from build123d import *

# Parameters (mm, degrees)
SKETCH1_R               = 4.25
BOSS_EXTRUDE1_DEPTH     = 2
SKETCH1_3_R             = 7.25
SKETCH1_3_R_2           = 4.25
BOSS_EXTRUDE2_DEPTH     = 12
CUT_EXTRUDE1_DEPTH      = 47.818799643
CUT_EXTRUDE1_DEPTH_BACK = 47.818799643
SKETCH2_R               = 1.5


with BuildPart() as part:
    # Sketch1 → Boss-Extrude1 (new body)
    with BuildSketch(Plane(origin=(0, 0, 0), x_dir=(1, 0, 0), z_dir=(0, 1, 0))):
        with BuildLine():
            Line((6.579861092, 3.044327186), (24.395183951, 20.859650045))
            Line((24.395183951, 20.859650045), (20.859650045, 24.395183951))
            Line((20.859650045, 24.395183951), (3.044327186, 6.579861092))
            ThreePointArc((3.044327186, 6.579861092), (2.774454885, 6.698126611), (2.5, 6.805328794))
            Line((2.5, 6.805328794), (2.5, 32))
            Line((2.5, 32), (-2.5, 32))
            Line((-2.5, 32), (-2.5, 6.805328794))
            ThreePointArc((-2.5, 6.805328794), (-2.774454885, 6.698126611), (-3.044327186, 6.579861092))
            Line((-3.044327186, 6.579861092), (-20.859650045, 24.395183951))
            Line((-20.859650045, 24.395183951), (-24.395183951, 20.859650045))
            Line((-24.395183951, 20.859650045), (-6.579861092, 3.044327186))
            ThreePointArc((-6.579861092, 3.044327186), (-6.698126611, 2.774454885), (-6.805328794, 2.5))
            Line((-6.805328794, 2.5), (-32, 2.5))
            Line((-32, 2.5), (-32, -2.5))
            Line((-32, -2.5), (-6.805328794, -2.5))
            ThreePointArc((-6.805328794, -2.5), (-6.698126611, -2.774454885), (-6.579861092, -3.044327186))
            Line((-6.579861092, -3.044327186), (-24.395183951, -20.859650045))
            Line((-24.395183951, -20.859650045), (-20.859650045, -24.395183951))
            Line((-20.859650045, -24.395183951), (-3.044327186, -6.579861092))
            ThreePointArc((-3.044327186, -6.579861092), (-2.774454885, -6.698126611), (-2.5, -6.805328794))
            Line((-2.5, -6.805328794), (-2.5, -32))
            Line((-2.5, -32), (2.5, -32))
            Line((2.5, -32), (2.5, -6.805328794))
            ThreePointArc((2.5, -6.805328794), (2.774454885, -6.698126611), (3.044327186, -6.579861092))
            Line((3.044327186, -6.579861092), (20.859650045, -24.395183951))
            Line((20.859650045, -24.395183951), (24.395183951, -20.859650045))
            Line((24.395183951, -20.859650045), (6.579861092, -3.044327186))
            ThreePointArc((6.579861092, -3.044327186), (6.698126611, -2.774454885), (6.805328794, -2.5))
            Line((6.805328794, -2.5), (32, -2.5))
            Line((32, -2.5), (32, 2.5))
            Line((32, 2.5), (6.805328794, 2.5))
            ThreePointArc((6.805328794, 2.5), (6.698126611, 2.774454885), (6.579861092, 3.044327186))
        make_face()
        with Locations(Location((0, 0, 0), (0, 0, 270))):
            Circle(SKETCH1_R, mode=Mode.SUBTRACT)
    extrude(amount=BOSS_EXTRUDE1_DEPTH)

    # Sketch1_3 → Boss-Extrude2 (add)
    with BuildSketch(Plane(origin=(0, 0, 0), x_dir=(1, 0, 0), z_dir=(0, 1, 0))):
        with Locations(Location((0, 0, 0), (0, 0, 69.828728654))):
            Circle(SKETCH1_3_R)
        with Locations(Location((0, 0, 0), (0, 0, 270))):
            Circle(SKETCH1_3_R_2, mode=Mode.SUBTRACT)
    extrude(amount=BOSS_EXTRUDE2_DEPTH)

    # Sketch2 → Cut-Extrude1 (cut, two sides: drawn at the far end of the back side and taken through both)
    with BuildSketch(Plane.XY.offset(-CUT_EXTRUDE1_DEPTH_BACK)):
        with Locations((0, 9)):
            Circle(SKETCH2_R)
    extrude(amount=CUT_EXTRUDE1_DEPTH + CUT_EXTRUDE1_DEPTH_BACK, mode=Mode.SUBTRACT)


solid = part.part
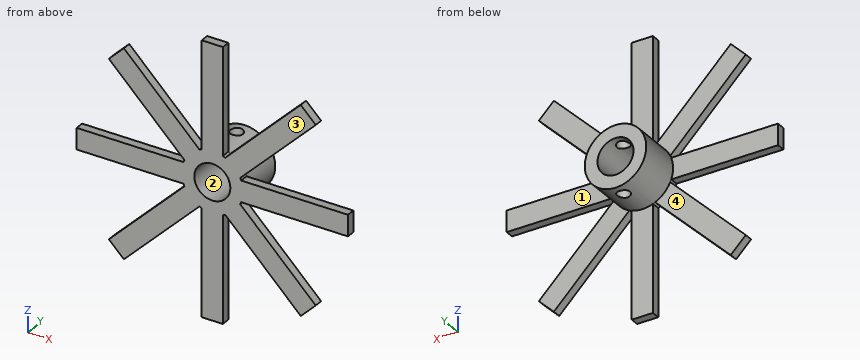
Model file for the job. Use its own axes, mm. Face numbers are marked on the shaded views. A direction names the side the tool comes from. Give positions to 0.01 mm unless a question says otherwise; leave off trailing zeros. Loops run counter-clockwise (first coordinate to the right, second up) from the corner with the lowest first, then second, coordinate; pieces in that order, holes last. Notation, with made-up numbers: (32, -10.75) -> (59, -10.75) arc R27 cw to (59, 14.25) -> close; hole circle Ø3 at (-20, 88.5). An arc over 180 degrees is marked (long way). Use a Markdown table: item, result. Add a question column.
(1) Slice it at A-A on x = 0. List the corners of the cut face in (y, z), and give its area (3 significant figures).
(2) Drop flat-ended pins along their axis: pin 1 Ø1 at (x, y) = (-22, 1) entering from -Z; pin 2 Ø0.6 at (x, y) = (-16.5, 0.5) entering from +Z; pin 3 Ø1.6 at (y, z) = (0.5, 20) entering from -X. Give the stop position or say it passes through.
(3) Slice it at B-B on y = 9. List the corners of the cut face in (x, z), and give its area (3 significant figures).
(4) Tool access for the marked faces 3 and 4: list every direction of +Z, -Z, +X, -X, +Y, -Y with a clear straight run to the whole face (end or side of a thin tool).
(5) Wall check: line 1 along Y through (x, z) = (0, 5); line 2 along Z through (x, y) = (-13.5, 1.5); line 3 along Z through (x, y) = (21.5, 1). Give the ranges that are in metal, low to high.
(6) Slice it at C-C on z = 0. List the corners of the cut face in (x, y), and give its area (3 significant figures).
(7) Mould opens along X. For the marked faces 1 and 2 say: +X half, -X half, draft (parallel to the pull), parting line (faces both ways), or undercut.
(8) Slice it at D-D on x = -17. List the corners of the cut face in (y, z), and give its area (3 significant figures).
Filled sheet:
| question | item | result |
|---|---|---|
| 1 | outline | (0, -32) -> (2, -32) -> (2, -7.25) -> (7.5, -7.25) -> (7.5, -4.25) -> (0, -4.25) -> close; (0, 4.25) -> (7.5, 4.25) -> (7.5, 7.25) -> (2, 7.25) -> (2, 32) -> (0, 32) -> close; (10.5, -7.25) -> (12, -7.25) -> (12, -4.25) -> (10.5, -4.25) -> close; (10.5, 4.25) -> (12, 4.25) -> (12, 7.25) -> (10.5, 7.25) -> close |
| 1 | area | 153 mm2 |
| 2 | pin 1 | z = -23.75 |
| 2 | pin 2 | z = 20.34 |
| 2 | pin 3 | x = -24.34 |
| 3 | outline | (-1.5, -7.09) -> (-1.5, -3.98) arc R4.25 cw to (-1.5, 3.98) -> (-1.5, 7.09) arc R7.25 ccw to start; (1.5, -7.09) arc R7.25 ccw to (1.5, 7.09) -> (1.5, 3.98) arc R4.25 cw to (1.5, -3.98) -> close |
| 3 | area | 90.2 mm2 |
| 4 | face 3 | +Z, -Z, +X, -X, -Y |
| 4 | face 4 | -Z, -X, +Y |
| 5 | line 1 | 0 to 7.5, 10.5 to 12 |
| 5 | line 2 | -17.04 to -9.96, -2.5 to 2.5, 9.96 to 17.04 |
| 5 | line 3 | -23.75 to -17.96, -2.5 to 2.5, 17.96 to 23.75 |
| 6 | outline | (-32, 0) -> (-4.25, 0) -> (-4.25, 12) -> (-7.25, 12) -> (-7.25, 2) -> (-32, 2) -> close; (4.25, 0) -> (32, 0) -> (32, 2) -> (7.25, 2) -> (7.25, 12) -> (4.25, 12) -> close |
| 6 | area | 171 mm2 |
| 7 | face 1 | draft |
| 7 | face 2 | undercut |
| 8 | outline | (0, -20.54) -> (2, -20.54) -> (2, -13.46) -> (0, -13.46) -> close; (0, -2.5) -> (2, -2.5) -> (2, 2.5) -> (0, 2.5) -> close; (0, 13.46) -> (2, 13.46) -> (2, 20.54) -> (0, 20.54) -> close |
| 8 | area | 38.3 mm2 |
